The model under review builds one solid part; all positions refer to its coordinate system, in mm. A direction names the side the tool comes from. Coordinates: 2 decimals unless noted, no trailing zeros. Write each loop counter-clockwise with the first axis right and the second up, starting at its lowest first coordinate (ties: lowest second). Pieces come first, ordered by that corner, then holes.
```python
from build123d import *

# Parameters (mm, degrees)
SKETCH_1_W             = 50
SKETCH_1_H             = 6
EXTRUDE_1_DEPTH        = 6
SKETCH_2_R             = 2.15
EXTRUDE_2_DEPTH        = 2.5
PATTERN_LINEAR_1_COUNT = 2
PATTERN_LINEAR_1_PITCH = 52.5


with BuildPart() as part:
    # 草圖1 → 填料-伸長1 (new body)
    with BuildSketch(Plane.XY):
        with Locations((25, 3)):
            Rectangle(SKETCH_1_W, SKETCH_1_H)
    extrude(amount=EXTRUDE_1_DEPTH)

    # 草圖2 → 填料-伸長2 (add)
    with BuildSketch(Plane.ZY):
        with Locations((3, 3)):
            Circle(SKETCH_2_R)
    extrude_2 = extrude(amount=EXTRUDE_2_DEPTH)

    # 直線複製排列1: 填料-伸長2 ×2
    with Locations(*[(i * PATTERN_LINEAR_1_PITCH, 0, 0) for i in range(1, PATTERN_LINEAR_1_COUNT)]):
        add(extrude_2)


solid = part.part
```
Item 1: To check wall thickness, follow line 1 along X through (y, z) = (5.55, 1). State the ranges of the line that lie inside material, in increasing order.
Solved:
line 1: x = 0 to 50
Item 2: Take a section at A-A, the plane y = 3. Write out the cut boundary in (x, z).
Solved:
outline: (-2.5, 0.85) - (0, 0.85) - (0, 0) - (50, 0) - (50, 0.85) - (52.5, 0.85) - (52.5, 5.15) - (50, 5.15) - (50, 6) - (0, 6) - (0, 5.15) - (-2.5, 5.15) - close
Item 3: Machinability: for faces 1 (the face through (-2.5, 3, 3)), 2 (the face through (51.27, 3.09, 0.85)), 3 (the face through (-1.23, 3.09, 0.85)), which of the approach directions +Z, -Z, +X, -X, +Y, -Y give a long, thin tool a straight path to every point of the face, cutting with its end or side? Answer none if there is none.
Solved:
face 1: +Z, -Z, -X, +Y, -Y
face 2: +X
face 3: -X
